Verification items for this drawing (mm, ordinates from the low corner). A direction names the side the tool comes from. Round coordinates to 2 decimals unless told otherwise and drop trailing zeros. Write each loop counter-clockwise with the first axis right and the second up, starting at its lowest first coordinate (ties: lowest second). Pieces come first, ordered by that corner, then holes. Notation, with made-up numbers: (11, 85.25) -> (66, 85.25) arc R9 cw to (66, 97.25) -> close; hole circle Ø6 at (-26.75, 73). An arc over 180 degrees is marked (long way). Use one line per item in the form item = value. Start each with the question number.
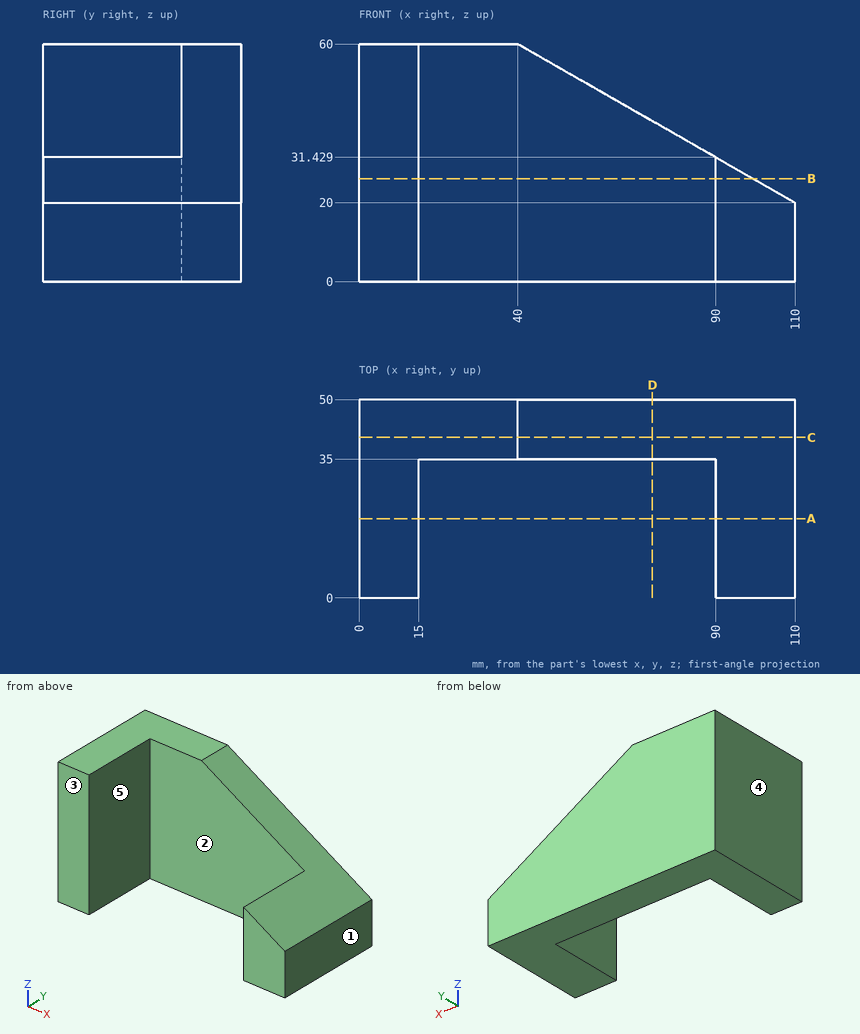
1. Mould release check, pull along X, two halves, no side actions. Record for the marked faces 1, 2 and 3: +X half, -X half, draft (parallel to the pull), parting line (faces both ways), or undercut.
2. Sectioned sample at D-D (x = 74). Enter the section's corners in (y, z).
3. Depth check by flat-ended pin: pin 1 (6 mm diameter, centred on y = 23, z = 37, fed in from +X); pin 2 (4 mm diameter, centred on x = 31, z = 9, fed in from -Y); pin 3 (1.5 mm diameter, centred on x = 52, y = 39, fed in from +Z). Enter the tip coordinate at first touch or a pass-through.
4. Tool access check on the marked faces 4 and 5. Record the directions out of +Z, -Z, +X, -X, +Y, -Y that give a thin tool (end or side, any length) a straight path to the whole face; none if there is none.
5. Sectioned sample at C-C (y = 40.5). Enter the section's corners in (x, z).
6. Sectioned sample at B-B (z = 26). Enter the section's corners in (x, y), and give its area (3 significant figures).
7. Sectioned sample at A-A (y = 20). Enter the section's corners in (x, z).
8. Scan lines: probe 1 along X at (y, z) = (26, 10.5); probe 2 along Y at (x, z) = (85.5, 18); probe 3 along X at (y, z) = (15, 58). Record each from-to range of solid material in increasing order.
Returned:
q1.face_1 = +X half
q1.face_2 = undercut
q1.face_3 = draft
q2.outline = (35, 0) -> (50, 0) -> (50, 40.57) -> (35, 40.57) -> close
q3.pin_1 = 15
q3.pin_2 = 35
q3.pin_3 = 53.57
q4.face_4 = +Z, -Z, -X, +Y, -Y
q4.face_5 = +Z, -Z, -Y
q5.outline = (0, 0) -> (110, 0) -> (110, 20) -> (40, 60) -> (0, 60) -> close
q6.outline = (0, 0) -> (15, 0) -> (15, 35) -> (90, 35) -> (90, 0) -> (99.5, 0) -> (99.5, 50) -> (0, 50) -> close
q6.area = 2,350 mm^2
q7.outline = (0, 0) -> (15, 0) -> (15, 60) -> (0, 60) -> close; (90, 0) -> (110, 0) -> (110, 20) -> (90, 31.43) -> close
q8.probe_1 = 0 to 15, 90 to 110
q8.probe_2 = 35 to 50
q8.probe_3 = 0 to 15
